```python
from build123d import *

# Parameters (mm, degrees)
F1_DEPTH = 115
F2_DEPTH = 5
F3_R     = 6
F4_R     = 4.5
F5_DEPTH = 4
F7_DEPTH = 4


with BuildPart() as f1:
    # F0 (on Top) → F1 (new body)
    with BuildSketch(Plane.XY):
        with BuildLine():
            ThreePointArc((-4.21e-08, -9.5), (6.7175144064, -6.7175144362), (9.5, 0))
            ThreePointArc((9.5, 0), (6.7175144305, 6.7175144121), (2.6e-08, 9.5))
            ThreePointArc((2.6e-08, 9.5), (-9.5, 3.4e-08), (-4.21e-08, -9.5))
        make_face()
    extrude(amount=F1_DEPTH)

    # F0 (on Top) → F2 (join)
    with BuildSketch(Plane.XY):
        with BuildLine():
            ThreePointArc((-4.21e-08, -9.5), (-9.5, 3.4e-08), (2.6e-08, 9.5))
            Line((2.6e-08, 9.5), (-25, 9.5))
            Line((-25, 9.5), (-25, -9.5))
            Line((-25, -9.5), (-4.21e-08, -9.5))
        make_face()
        with BuildLine():
            ThreePointArc((2.6e-08, 9.5), (6.7175144305, 6.7175144121), (9.5, 0))
            ThreePointArc((9.5, 0), (6.7175144064, -6.7175144362), (-4.21e-08, -9.5))
            Line((-4.21e-08, -9.5), (25, -9.5))
            Line((25, -9.5), (25, 9.5))
            Line((25, 9.5), (2.6e-08, 9.5))
        make_face()
        with BuildLine():
            ThreePointArc((-4.21e-08, -9.5), (6.7175144064, -6.7175144362), (9.5, 0))
            ThreePointArc((9.5, 0), (6.7175144305, 6.7175144121), (2.6e-08, 9.5))
            ThreePointArc((2.6e-08, 9.5), (-9.5, 3.4e-08), (-4.21e-08, -9.5))
        make_face()
    extrude(amount=-F2_DEPTH)

    # F3
    f3_edges = [f1.edges().sort_by_distance(p)[0] for p in [
        (-25, 9.5, -2.5),
        (-25, -9.5, -2.5),
        (25, 9.5, -2.5),
        (25, -9.5, -2.5),
    ]]
    fillet(f3_edges, radius=F3_R)

    # F4 (on face) → F5 (join)
    with BuildSketch(Plane.XY.offset(115)):
        Circle(F4_R)
    extrude(amount=F5_DEPTH)

    # F6 (on face) → F7 (join)
    with BuildSketch(Plane.XY.offset(119)):
        with BuildLine():
            ThreePointArc((4.5, 0), (3.1819805153, 3.1819805153), (0, 4.5))
            ThreePointArc((0, 4.5), (-4.5, 0), (0, -4.5))
            ThreePointArc((0, -4.5), (3.1819805153, -3.1819805153), (4.5, 0))
        make_face()
        with BuildLine():
            Line((0, 4.5), (-8.3666002653, 4.5))
            ThreePointArc((-8.3666002653, 4.5), (-9.2122934854, 2.3202691093), (-9.5, 0))
            ThreePointArc((-9.5, 0), (-9.2122934854, -2.3202691093), (-8.3666002653, -4.5))
            Line((-8.3666002653, -4.5), (0, -4.5))
            ThreePointArc((0, -4.5), (-4.5, 0), (0, 4.5))
        make_face()
        with BuildLine():
            Line((8.3666002653, 4.5), (0, 4.5))
            ThreePointArc((0, 4.5), (3.1819805153, 3.1819805153), (4.5, 0))
            ThreePointArc((4.5, 0), (3.1819805153, -3.1819805153), (0, -4.5))
            Line((0, -4.5), (8.3666002653, -4.5))
            ThreePointArc((8.3666002653, -4.5), (9.2122934854, -2.3202691093), (9.5, 0))
            ThreePointArc((9.5, 0), (9.2122934854, 2.3202691093), (8.3666002653, 4.5))
        make_face()
    extrude(amount=F7_DEPTH)


solid = f1.part
```
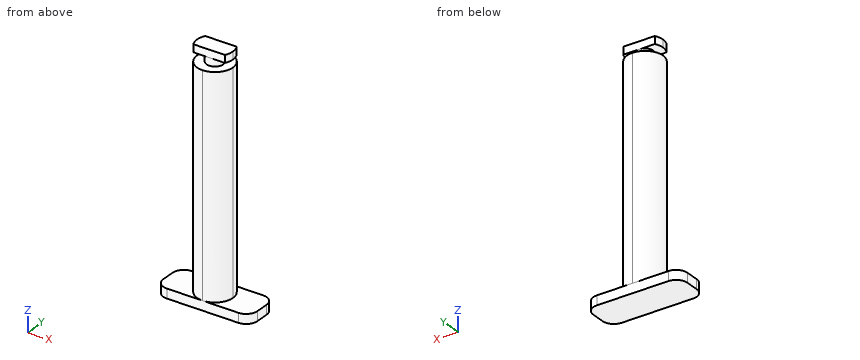
Part model, mm, in its own coordinate system. Coordinates: 2 decimals unless noted, no trailing zeros. Write each loop counter-clockwise with the first axis right and the second up, starting at its lowest first coordinate (ties: lowest second). Pieces come first, ordered by that corner, then holes.
Item 1: Slice it at C-C (x = 16). Write the cut outline in (y, z), and give its area (3 significant figures).
Item 2: Slice it at B-B (y = -7). Write the cut outline in (x, z).
Item 3: Slice it at A-A (z = 56). Write the cut outline in (x, y).
Item 4: Probe line 1 (Z direction, x = -8, y = -8); line 2 (Z direction, x = 4, y = 4.75); line 3 (Y direction, x = 0.5, z = 5). List the from-to ranges inside material, lowest first.
Item 5: Slice it at D-D (y = -2). Write the cut outline in (x, z), and give its area (3 significant figures).
Item 6: Pin check, flat tips, straight feed: pin 1 (1.2 mm diameter, centred on x = -4, z = 121.5, fed in from +Y); pin 2 (1.2 mm diameter, centred on x = -0.5, z = 121.5, fed in from -Y); pin 3 (10 mm diameter, centred on y = 1.5, z = 78, fed in from +X); pin 4 (10 mm diameter, centred on x = -15, z = 40.5, fed in from +Y). Stop position of each tip, or through.
Results found:
1. outline: (-9.5, -5) - (9.5, -5) - (9.5, 0) - (-9.5, 0) - close
1. area: 95.0 mm2
2. outline: (-23.87, -5) - (23.87, -5) - (23.87, 0) - (6.42, 0) - (6.42, 115) - (-6.42, 115) - (-6.42, 0) - (-23.87, 0) - close
3. outline: circle Ø19 at (0, 0)
4. line 1: z = -5 to 0
4. line 2: z = -5 to 115
4. line 3: y = -9.49 to 9.49
5. outline: (-25, -5) - (25, -5) - (25, 0) - (9.29, 0) - (9.29, 115) - (4.03, 115) - (4.03, 119) - (9.29, 119) - (9.29, 123) - (-9.29, 123) - (-9.29, 119) - (-4.03, 119) - (-4.03, 115) - (-9.29, 115) - (-9.29, 0) - (-25, 0) - close
5. area: 2,490 mm2
6. pin 1: stops at y = 4.5
6. pin 2: stops at y = -4.5
6. pin 3: stops at x = 9.5
6. pin 4: passes through
